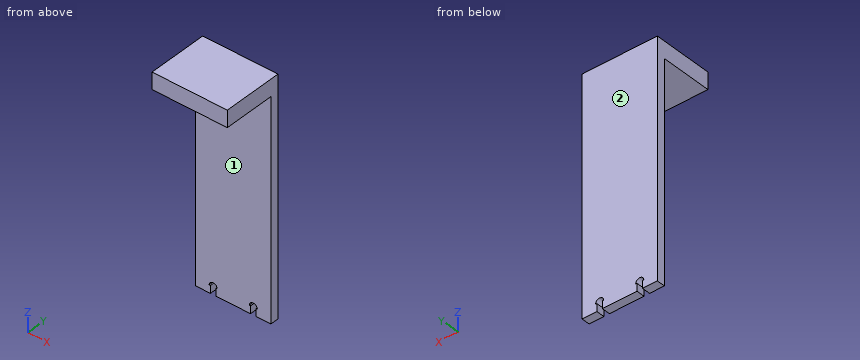
```python
from build123d import *

# Parameters (mm, degrees)
BOSS_EXTRUDE1_DEPTH = 2.5
SKETCH4_W           = 54.285
SKETCH4_H           = 130
CUT_EXTRUDE1_DEPTH  = 120
SKETCH5_W           = 10
SKETCH5_H           = 35.9
BOSS_EXTRUDE2_DEPTH = 22.5


with BuildPart() as part:
    # Sketch2 → Boss-Extrude1 (new, symmetric)
    with BuildSketch(Plane(origin=(0, 0, 0), x_dir=(1, 0, 0), z_dir=(0, 1, 0))):
        with BuildLine():
            Line((-13.65, 65), (-76.785, 65))
            Line((-76.785, 65), (-76.785, -65))
            Line((-76.785, -65), (76.785, -65))
            Line((76.785, -65), (76.785, 65))
            Line((76.785, 65), (13.65, 65))
            Line((13.65, 65), (13.65, 60.5))
            Line((13.65, 60.5), (14.4, 60.5))
            ThreePointArc((14.4, 60.5), (12, 58.1), (9.6, 60.5))
            Line((9.6, 60.5), (10.35, 60.5))
            Line((10.35, 60.5), (10.35, 65))
            Line((10.35, 65), (-10.35, 65))
            Line((-10.35, 65), (-10.35, 60.5))
            Line((-10.35, 60.5), (-9.6, 60.5))
            ThreePointArc((-9.6, 60.5), (-12, 58.1), (-14.4, 60.5))
            Line((-14.4, 60.5), (-13.65, 60.5))
            Line((-13.65, 60.5), (-13.65, 65))
        make_face()
    extrude(amount=BOSS_EXTRUDE1_DEPTH, both=True)

    # Sketch4 → Cut-Extrude1 (cut)
    with BuildSketch(Plane(origin=(0, 2.5, 0), x_dir=(1, 0, 0), z_dir=(0, 1, 0))):
        with Locations((-49.6425, 0)):
            Rectangle(SKETCH4_W, SKETCH4_H)
        with Locations((49.6425, 0)):
            Rectangle(SKETCH4_W, SKETCH4_H)
    extrude(amount=-CUT_EXTRUDE1_DEPTH, mode=Mode.SUBTRACT)

    # Sketch5 → Boss-Extrude2 (add, symmetric)
    with BuildSketch(Plane(origin=(0, 0, 0), x_dir=(0, 0, -1), z_dir=(1, 0, 0))):
        with Locations((-70, -15.45)):
            Rectangle(SKETCH5_W, SKETCH5_H)
    extrude(amount=BOSS_EXTRUDE2_DEPTH, both=True)


solid = part.part
```
Check sheet for the modelled part. Datum: model origin and axes. Units: mm. Face numbers are marked on the shaded views. A direction names the side the tool comes from. Round coordinates to 2 decimals unless told otherwise and drop trailing zeros. Loops run counter-clockwise (first coordinate to the right, second up) from the corner with the lowest first, then second, coordinate; pieces in that order, holes last. Notation, with made-up numbers: (12.5, 87.25) -> (62.5, 87.25) arc R11 cw to (62.5, 101.25) -> close; hole circle Ø4 at (58.25, 6.5). An arc over 180 degrees is marked (long way). Answer in a Markdown table with one row per item.
Q1. Set-up check for the marked faces 1 and 2: record each of +Z, -Z, +X, -X, +Y, -Y from which the full face is reachable in a straight line by a thin tool's end or side.
Data:
| item | result |
|---|---|
| face 1 | -Z, +X, -X, -Y |
| face 2 | +Z, -Z, +X, -X, +Y |
Q2. Thickness scan on L1, parallel to Z at x = -3, y = -17; L2, parallel to Y at x = -3, z = -15. Record the ranges inside material, lowest first.
Data:
| item | result |
|---|---|
| L1 | z = 65 to 75 |
| L2 | y = -2.5 to 2.5 |
Q3. Sectioned sample at B-B on z = 19. Enter the section's corners in (x, y).
Data:
| item | result |
|---|---|
| outline | (-22.5, -2.5) -> (22.5, -2.5) -> (22.5, 2.5) -> (-22.5, 2.5) -> close |
Q4. Sectioned sample at A-A on x = 12. Enter the section's corners in (y, z).
Data:
| item | result |
|---|---|
| outline | (-33.4, 65) -> (-2.5, 65) -> (-2.5, -58.1) -> (2.5, -58.1) -> (2.5, 75) -> (-33.4, 75) -> close |
Q5. Sectioned sample at C-C on y = -16. Enter the section's corners in (x, z), then the cut area to 3 significant figures.
Data:
| item | result |
|---|---|
| outline | (-22.5, 65) -> (22.5, 65) -> (22.5, 75) -> (-22.5, 75) -> close |
| area | 450 mm^2 |
Q6. Go/stop test with flat-tipped pins: P1, Ø6, axis at x = -17, z = 40, coming from the -Y side; P2, Ø12, axis at x = -15.5, y = -25.5, coming from the -Z side. Record where each tip stops, or that it passes through.
Data:
| item | result |
|---|---|
| P1 | stops at y = -2.5 |
| P2 | stops at z = 65 |
